Verification items for the finished model (mm, model axes). Face numbers are marked on the shaded views. A direction names the side the tool comes from. Coordinates: 2 decimals unless noted, no trailing zeros. Write each loop counter-clockwise with the first axis right and the second up, starting at its lowest first coordinate (ties: lowest second). Pieces come first, ordered by that corner, then holes. Notation, with made-up numbers: (77, -0.5) -> (124, -0.5) arc R16 cw to (124, 20.5) -> close; hole circle Ø11 at (80, 21). An arc over 180 degrees is marked (long way). Answer in a Markdown table with one row per item.
```python
from build123d import *

# Parameters (mm, degrees)
EXTRUDE_1_DEPTH     = 62.96
SKETCH_2_W          = 28.8
SKETCH_2_H          = 2
EXTRUDE_2_DEPTH     = 22
SKETCH_7_W          = 1.8
SKETCH_7_H          = 45.791930202
CUT_EXTRUDE_1_DEPTH = 22
FILLET_2_R          = 5
MM_PRESS_3_D        = 3
SKETCH_14_W         = 28.8
SKETCH_14_H         = 2.5
EXTRUDE_3_DEPTH     = 30
FILLET_3_R          = 6
FILLET_4_R          = 5


with BuildPart() as part:
    # 草图1 → 凸台-拉伸1 (new body)
    with BuildSketch(Plane.XY):
        Polygon((-13.750151713, 26.893062898), (-13.750151713, 1.893062898), (15.049848287, 1.893062898), (15.049848287, 26.893062898), (12.049848287, 26.893062898), (12.049848287, 4.893062898), (-10.750151713, 4.893062898), (-10.750151713, 26.893062898), align=None)
    extrude(amount=EXTRUDE_1_DEPTH)

    # 草图2 → 凸台-拉伸2 (add)
    with BuildSketch(Plane(origin=(0, 4.893062898, 0), x_dir=(1, 0, 0), z_dir=(0, 1, 0))):
        with Locations((0.649848287, -1)):
            Rectangle(SKETCH_2_W, SKETCH_2_H)
    extrude(amount=EXTRUDE_2_DEPTH)

    # 草图7 → 切除-拉伸1 (cut)
    with BuildSketch(Plane(origin=(0, 4.893062898, 0), x_dir=(1, 0, 0), z_dir=(0, 1, 0))):
        with Locations((-11.650151713, -31.026293471)):
            Rectangle(SKETCH_7_W, SKETCH_7_H)
        with Locations((12.949848287, -31.026293471)):
            Rectangle(SKETCH_7_W, SKETCH_7_H)
    extrude(amount=CUT_EXTRUDE_1_DEPTH, mode=Mode.SUBTRACT)

    # 圆角2
    fillet_2_edges = [part.edges().sort_by_distance(p)[0] for p in [
        (0.649848287, 4.893062898, 2),
    ]]
    fillet(fillet_2_edges, radius=FILLET_2_R)

    # 大小mm Press 暗销孔3 (through all)
    with Locations(Plane(origin=(15.049848287, 207.544632648, -30.881320252), x_dir=(0, -0.022253058, 0.99975237), z_dir=(1, 0, 0))):
        with Locations((93.161367469, 190.578219389), (93.161367469, 182.547127137), (40.245392963, 190.578219389), (40.245392963, 182.547127137)):
            Hole(MM_PRESS_3_D / 2)

    # 草图14 → 凸台-拉伸3 (add)
    with BuildSketch(Plane(origin=(0, 4.893062898, 0), x_dir=(1, 0, 0), z_dir=(0, 1, 0))):
        with Locations((0.649848287, -61.71)):
            Rectangle(SKETCH_14_W, SKETCH_14_H)
    extrude(amount=EXTRUDE_3_DEPTH)

    # 圆角3
    fillet_3_edges = [part.edges().sort_by_distance(p)[0] for p in [
        (0.649848287, 4.893062898, 60.46),
    ]]
    fillet(fillet_3_edges, radius=FILLET_3_R)

    # 圆角4
    fillet_4_edges = [part.edges().sort_by_distance(p)[0] for p in [
        (13.549848287, 26.893062898, 60.46),
        (-12.250151713, 26.893062898, 60.46),
    ]]
    fillet(fillet_4_edges, radius=FILLET_4_R)


solid = part.part
```
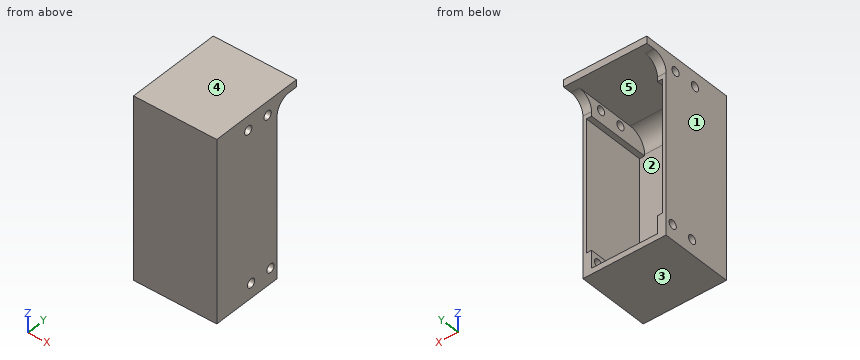
1. Material ranges on probe 1 along X at (y, z) = (18, 14.5); probe 2 along X at (y, z) = (21, 4); probe 3 along Z at (x, y) = (7.5, 18), recorded low to high. Write a range as from..to.
Findings below:
| item | result |
|---|---|
| probe 1 | x = -13.75..-12.55, 13.85..15.05 |
| probe 2 | x = -13.75..-10.75, 12.05..15.05 |
| probe 3 | z = 0..2, 60.46..62.96 |
2. Release check for a two-part mould opening along X. For the marked faces 1, 2 and 3 record: released by +X, released by -X, zero draft, split by the parting line, or undercut.
Findings below:
| item | result |
|---|---|
| face 1 | released by -X |
| face 2 | undercut |
| face 3 | zero draft |
3. Sectioned sample at B-B, the plane z = 33. Record the cut outline in (x, y), and give its area (3 significant figures).
Findings below:
| item | result |
|---|---|
| outline | (-13.75, 1.89) -> (15.05, 1.89) -> (15.05, 26.89) -> (13.85, 26.89) -> (13.85, 4.89) -> (-12.55, 4.89) -> (-12.55, 26.89) -> (-13.75, 26.89) -> close |
| area | 139 mm² |
4. Sectioned sample at A-A, the plane z = 58. Record the cut outline in (x, y), and give its area (3 significant figures).
Findings below:
| item | result |
|---|---|
| outline | (-13.75, 1.89) -> (15.05, 1.89) -> (15.05, 13.44) -> (12.05, 13.44) -> (12.05, 6.05) -> (-10.75, 6.05) -> (-10.75, 13.44) -> (-13.75, 13.44) -> close; (-13.75, 16.44) -> (-10.75, 16.44) -> (-10.75, 21.48) -> (-13.75, 21.48) -> close; (-13.75, 24.46) -> (-10.75, 24.46) -> (-10.75, 27.59) -> (-13.75, 27.59) -> close; (12.05, 16.44) -> (15.05, 16.44) -> (15.05, 21.48) -> (12.05, 21.48) -> close; (12.05, 24.46) -> (15.05, 24.46) -> (15.05, 27.59) -> (12.05, 27.59) -> close |
| area | 213 mm² |
5. Sectioned sample at C-C, the plane x = -9.25. Record the cut outline in (y, z).
Findings below:
| item | result |
|---|---|
| outline | (1.89, 0) -> (26.89, 0) -> (26.89, 2) -> (9.89, 2) arc R5 cw to (4.89, 7) -> (4.89, 54.46) arc R6 cw to (10.89, 60.46) -> (34.89, 60.46) -> (34.89, 62.96) -> (1.89, 62.96) -> close |
6. Sectioned sample at D-D, the plane y = 6.5. Record the cut outline in (x, z).
Findings below:
| item | result |
|---|---|
| outline | (-13.75, 0) -> (15.05, 0) -> (15.05, 62.96) -> (-13.75, 62.96) -> close; hole (-12.55, 8.13) -> (-10.75, 8.13) -> (-10.75, 3.33) -> (12.05, 3.33) -> (12.05, 8.13) -> (13.85, 8.13) -> (13.85, 53.92) -> (12.05, 53.92) -> (12.05, 58.55) -> (-10.75, 58.55) -> (-10.75, 53.92) -> (-12.55, 53.92) -> close |
7. Access from +Z, -Z, +X, -X, +Y, -Y to the whole of each face (thin tool, end or side, straight path). Record for the marked faces 4 and 5.
Findings below:
| item | result |
|---|---|
| face 4 | +Z, +X, -X, +Y, -Y |
| face 5 | +Y |
8. Go/stop test with a flat-tipped pin: pin 1 (14.5 mm diameter, centred on x = 6, z = 37, fed in from +Y). Record where the tip stops, or that it passes through.
Findings below:
| item | result |
|---|---|
| pin 1 | stops at y = 4.89 |
